Can you work these out from the model? Positions are in its coordinate system, mm. A direction names the side the tool comes from. Give positions to 0.01 mm unless a question says otherwise; leave off trailing zeros. Order: outer loops, then holes, each group sorted by start corner. A loop starts at its lowest first (then second) coordinate and runs counter-clockwise, first axis right, second up. Notation, with made-up numbers: (-26.5, 6.25) - (-16.5, 6.25) arc R10 ccw to (-16.5, 22.25) - close; hole circle Ø6 at (26, 80). An arc over 180 degrees is marked (long way). Return JSON: item names as keys, results as strings.
```python
from build123d import *

# Parameters (mm, degrees)
SKETCH1_W                = 9.5
SKETCH1_H                = 59
BOSS_EXTRUDE1_DEPTH      = 9.5
SKETCH2_R                = 7.45
BOSS_EXTRUDE2_DEPTH      = 19
BOSS_EXTRUDE2_DEPTH_BACK = 9.5
BOSS_EXTRUDE3_DEPTH      = 8


with BuildPart() as part:
    # Sketch1 → Boss-Extrude1 (new body)
    with BuildSketch(Plane(origin=(0, 0, 0), x_dir=(1, 0, 0), z_dir=(0, 1, 0))):
        Rectangle(SKETCH1_W, SKETCH1_H)
    extrude(amount=BOSS_EXTRUDE1_DEPTH)

    # Sketch2 → Boss-Extrude2 (add, two sides)
    with BuildSketch(Plane(origin=(0, 9.5, 0), x_dir=(1, 0, 0), z_dir=(0, 1, 0))) as boss_extrude2_sk:
        with Locations((0, -29.5)):
            Circle(SKETCH2_R)
    extrude(amount=BOSS_EXTRUDE2_DEPTH)
    extrude(boss_extrude2_sk.sketch, amount=-BOSS_EXTRUDE2_DEPTH_BACK)

    # Sketch3 → Boss-Extrude3 (add)
    with BuildSketch(Plane(origin=(0, 28.5, 0), x_dir=(1, 0, 0), z_dir=(0, 1, 0))):
        with BuildLine():
            Line((-1.3, -25.929285786), (-1.3, -24.329285786))
            Line((-1.3, -24.329285786), (1.3, -24.329285786))
            Line((1.3, -24.329285786), (1.3, -25.929285786))
            ThreePointArc((1.3, -25.929285786), (2.687005769, -26.812994231), (3.570714214, -28.2))
            Line((3.570714214, -28.2), (5.170714214, -28.2))
            Line((5.170714214, -28.2), (5.170714214, -30.8))
            Line((5.170714214, -30.8), (3.570714214, -30.8))
            ThreePointArc((3.570714214, -30.8), (-2.687005769, -32.187005769), (-1.3, -25.929285786))
        make_face()
    extrude(amount=BOSS_EXTRUDE3_DEPTH)


solid = part.part
```
1. If I drill on L1, parallel to Y at x = -1.25, z = -14.5; L2, parallel to Y at x = -0.75, z = 22.5; L3, parallel to X at y = 4.5, z = -26, over which ranges is the centre line in solid material (lowest first)? Write a range as [from, to].
Checks:
{"L1": "[0, 9.5]", "L2": "[0, 28.5]", "L3": "[-4.75, 4.75]"}
2. Suppose I cut it at A-A (x = 0). List the corners of the cut face in (y, z) for me.
Checks:
{"outline": "(0, -29.5) - (9.5, -29.5) - (9.5, 22.05) - (28.5, 22.05) - (28.5, 24.33) - (36.5, 24.33) - (36.5, 33.3) - (28.5, 33.3) - (28.5, 36.95) - (0, 36.95) - close"}
3. Suppose I cut it at B-B (y = 32). List the corners of the cut face in (x, z) for me.
Checks:
{"outline": "(-1.3, 24.33) - (1.3, 24.33) - (1.3, 25.93) arc R3.8 ccw to (3.57, 28.2) - (5.17, 28.2) - (5.17, 30.8) - (3.57, 30.8) arc R3.8 ccw (long way) to (-1.3, 25.93) - close"}
4. Suppose I cut it at D-D (y = 26). List the corners of the cut face in (x, z) for me.
Checks:
{"outline": "circle Ø14.9 at (0, 29.5)"}
5. On a 3-axis mill with a long thin cutter (end or side, diameter ignored), from which of +Z, -Z, +X, -X, +Y, -Y can I reach the whole of each face in a straight line? I mean faces 1 (the face through (5.171, 32, 29)), 2 (the face through (4, 32, 30.8)), 3 (the face through (-2.61, 32.44, 32.26)). Say none if no direction works.
Checks:
{"face 1": "+Z, -Z, +X, +Y", "face 2": "+Z, +X, +Y", "face 3": "+Y"}
6. For pin 1 Ø3 at (x, z) = (-4, -22.5) entering from +Y; pin 2 Ø10 at (y, z) = (16.5, 2) entering from -X; pin 3 Ø3 at (x, y) = (0, 34) entering from -Z; pin 4 Ø5 at (x, y) = (-4.5, 27) entering from +Z, each with a flat end and sliding along its axis, tell me the tip position at first contact or that it passes through.
Checks:
{"pin 1": "y = 9.5", "pin 2": "through", "pin 3": "z = 24.33", "pin 4": "z = 36.68"}
7. Suppose I cut it at C-C (z = -6). List the corners of the cut face in (x, y) for me, plus the area to 4 significant figures.
Checks:
{"outline": "(-4.75, 0) - (4.75, 0) - (4.75, 9.5) - (-4.75, 9.5) - close", "area": "90.25 mm^2"}
